Autodesk Inventor part; units mm, degrees
ref_plane "YZ Plane" through (0, 0, 0) normal (1, 0, 0) x (0, 1, 0)
ref_plane "XZ Plane" through (0, 0, 0) normal (0, 1, 0) x (-1, 0, 0)
ref_plane "XY Plane" through (0, 0, 0) normal (0, 0, 1) x (1, 0, 0)
sketch "Sketch1" plane through (0, 0, 0) normal (0, 1, 0) x (-1, 0, 0)
  line L0 (3.6662, -6.35) -> (-3.6662, -6.35)
  line L1 (-3.6662, -6.35) -> (-7.3323, 0)
  line L2 (-7.3323, 0) -> (-3.6662, 6.35)
  line L3 (-3.6662, 6.35) -> (3.6662, 6.35)
  line L4 (3.6662, 6.35) -> (7.3323, 0)
  line L5 (7.3323, 0) -> (3.6662, -6.35)
  point P0 (0, 0)
  point P1 (0, 0)
  dimension "d0" = 12.7
extrude "Extrusion1" add sketch "Sketch1" against normal blind 25.4
sketch "Sketch2" plane through (0, 0, 0) normal (0, 1, 0) x (1, 0, 0)
  circle A0 centre (0, 0) radius 4.7625
  dimension "d3" = 9.525
extrude "Extrusion2" add sketch "Sketch2" along normal blind 46.0375
sketch "Sketch3" plane through (0, -25.4, 0) normal (0, -1, 0) x (1, 0, 0)
  circle A0 centre (0, 0) radius 4.7625
  circle A1 centre (0, 0) radius 1.905
  dimension "d7" = 3.81
extrude "Extrusion3" cut sketch "Sketch3" against normal blind 25.4 contours A1
properties part number "Roller shaft" material "Aluminum 6061"
Verification items for the finished model (mm, model axes). A direction names the side the tool comes from. Give positions to 0.01 mm unless a question says otherwise; leave off trailing zeros. Order: outer loops, then holes, each group sorted by start corner. A loop starts at its lowest first (then second) coordinate and runs counter-clockwise, first axis right, second up. Notation, with made-up numbers: (2.25, -33) -> (16.25, -33) arc R37 cw to (16.25, 3) -> close; hole circle Ø5 at (82.25, 50.5). An arc over 180 degrees is marked (long way). Use a Markdown table: item, result.
1) Section check A-A, the plane y = -15. Record the boundary of the cut face in (x, z) (3 decimals).
Results:
| item | result |
|---|---|
| outline | (-7.332, 0) -> (-3.666, -6.35) -> (3.666, -6.35) -> (7.332, 0) -> (3.666, 6.35) -> (-3.666, 6.35) -> close; hole circle Ø3.81 at (0, 0) |
2) Material ranges on probe 1 along Z at (x, y) = (0, -13.25) (3 decimals); probe 2 along X at (y, z) = (-17, 1.75); probe 3 along Y at (x, z) = (5, 0.75), recorded low to high.
Results:
| item | result |
|---|---|
| probe 1 | -6.35 to -1.905, 1.905 to 6.35 |
| probe 2 | -6.32 to -0.75, 0.75 to 6.32 |
| probe 3 | -25.4 to 0 |
3) Section check D-D, the plane y = 18.5. Record the boundary of the cut face in (x, z) (1 decimal), then the cut area to 3 significant figures.
Results:
| item | result |
|---|---|
| outline | circle Ø9.5 at (0, 0) |
| area | 71.3 mm² |
4) Tool access check on faces 1 (the cylindrical face through (-3.78, 22.7, -2.9)), 2 (the flat face through (0, -13, -6.35)), 3 (the flat face through (0, 0, 0)). Record the directions out of +Z, -Z, +X, -X, +Y, -Y that give a thin tool (end or side, any length) a straight path to the whole face; none if there is none.
Results:
| item | result |
|---|---|
| face 1 | +Y |
| face 2 | -Z, +X, -X, +Y, -Y |
| face 3 | -Y |
5) Section check C-C, the plane z = 3.5. Record the boundary of the cut face in (x, y), then the cut area to 3 significant figures.
Results:
| item | result |
|---|---|
| outline | (-5.31, -25.4) -> (5.31, -25.4) -> (5.31, 0) -> (3.23, 0) -> (3.23, 46.04) -> (-3.23, 46.04) -> (-3.23, 0) -> (-5.31, 0) -> close |
| area | 567 mm² |
6) Depth check by flat-ended pin: pin 1 Ø1 at (y, z) = (5.5, -0.5) entering from +X; pin 2 Ø5 at (y, z) = (9.5, -3) entering from +X; pin 3 Ø3 at (y, z) = (-11, 1) entering from +X. Enter the tip coordinate at first touch or a pass-through.
Results:
| item | result |
|---|---|
| pin 1 | x = 4.76 |
| pin 2 | x = 4.74 |
| pin 3 | x = 7.33 |
